```python
from build123d import *

# Parameters (mm, degrees)
F1_DEPTH = 60
F2_W     = 3
F2_H     = 3
F3_DEPTH = 60
F4_DEPTH = 42


with BuildPart() as f1:
    # F0 (on Front) → F1 (new body)
    with BuildSketch(Plane.XZ):
        with BuildLine():
            Line((-6, 0), (0, 0))
            Line((0, 0), (0, 3))
            Line((0, 3), (-6.3828637444, 3.5))
            ThreePointArc((-6.3828637444, 3.5), (-7.5200895217, 3.1043228005), (-8, 2))
            ThreePointArc((-8, 2), (-7.4142135624, 0.5857864376), (-6, 0))
        make_face()
    extrude(amount=F1_DEPTH)

    # F2 (on face) → F3 (join)
    with BuildSketch(Plane.XZ.offset(60)):
        with Locations((1.5, 1.5)):
            Rectangle(F2_W, F2_H)
    extrude(amount=-F3_DEPTH)

    # F4 (cut): a face of the model
    f4_faces = [f1.faces().sort_by_distance(p)[0] for p in [
        (-2.4940313384, -60, 1.6228930979),
    ]]
    extrude(f4_faces, amount=-F4_DEPTH, mode=Mode.SUBTRACT)


solid = f1.part
```
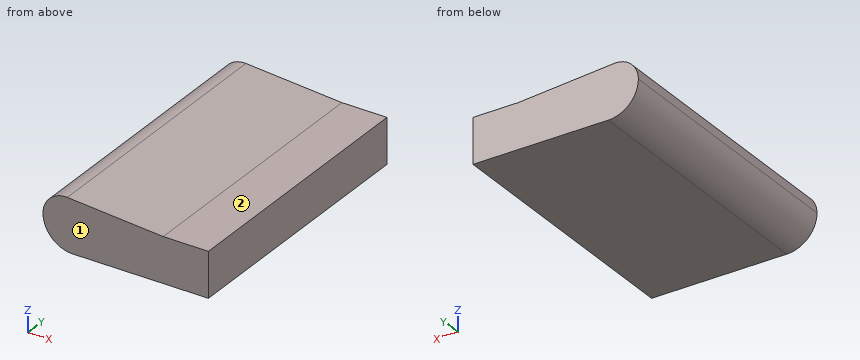
Work out the finished part from the listing and answer in its coordinate system (mm). Face numbers are marked on the shaded views. A direction names the side the tool comes from. Round coordinates to 2 decimals unless told otherwise and drop trailing zeros. Write each loop counter-clockwise with the first axis right and the second up, starting at its lowest first coordinate (ties: lowest second). Pieces come first, ordered by that corner, then holes. Notation, with made-up numbers: (-30, 28) -> (-22, 28) arc R28 cw to (-22, 53) -> close; hole circle Ø6 at (-23, -1). An arc over 180 degrees is marked (long way). Write each question's results on one line, items separated by ' | '.
1) The part is cut by section A-A (y = -9). Write down the section's boundary in (x, z), and give its area (3 significant figures).
Findings:
outline: (-8, 2) arc R2 ccw to (-6, 0) -> (3, 0) -> (3, 3) -> (0, 3) -> (-6.38, 3.5) arc R1.5 ccw to start | area: 34.1 mm²
2) Consider line 1 along Z through (x, y) = (0, -6); line 2 along X through (y, z) = (-4.5, 0.8); line 3 along Z through (x, y) = (-6.75, -4.75). Determine where each line is inside the solid, lowest interval first. Write a range as [from, to].
Findings:
line 1: z = [0, 3] | line 2: x = [-7.6, 3] | line 3: z = [0.15, 3.48]
3) Flat-ended cylindrical pins translate along their axes: pin 1 (5 mm diameter, centred on x = -6, y = -14.5, fed in from +Z); pin 2 (3.5 mm diameter, centred on x = 1.5, y = -8, fed in from +Z). Find the tip coordinate at first contact, or state that the pin passes through.
Findings:
pin 1: stops at z = 3.5 | pin 2: stops at z = 3.02
4) The part is cut by section C-C (z = 0.9). Write down the section's boundary in (x, y), and give its area (3 significant figures).
Findings:
outline: (-7.67, -18) -> (3, -18) -> (3, 0) -> (-7.67, 0) -> close | area: 192 mm²
5) The part is cut by section B-B (x = 2). Write down the section's boundary in (y, z).
Findings:
outline: (-18, 0) -> (0, 0) -> (0, 3) -> (-18, 3) -> close
6) Which of the six approach directions +Z, -Z, +X, -X, +Y, -Y give full straight-line access (tool end or side, diameter ignored) to the marked faces 1 and 2?
Findings:
face 1: +Z, -Z, +X, -X, -Y | face 2: +Z, +X, +Y, -Y
